CAD build for the part. Positions are in the model's coordinates, mm. A direction names the side the tool comes from. Coordinates: 2 decimals unless noted, no trailing zeros. Loops run counter-clockwise (first coordinate to the right, second up) from the corner with the lowest first, then second, coordinate; pieces in that order, holes last.
1) Pin check, flat tips, straight feed: pin 1 Ø0.8 at (y, z) = (0.5, 18) entering from -X; pin 2 Ø1.3 at (y, z) = (1, 6.5) entering from +X; pin 3 Ø0.8 at (x, y) = (-6, 1) entering from +Z. Stop position of each tip, or through.
2) Two-plate mould, pull along Y, no slides. Class faces 1 (the cylindrical face through (-21.197, -7.24, 12.522)), 2 (the flat face through (-21.374, 1, 19)), 3 (the cylindrical face through (-5.85, -8.62, 12.52)), 4 (the flat face through (-6, 1.588, 6)): +Y half, -Y half, draft (parallel to the pull), parting line (faces both ways), or undercut.
3) Saw through at C-C, the plane y = -6.35. Write the cut outline in (x, z).
4) Which spindle directions (+Z, -Z, +X, -X, +Y, -Y) get a long thin tool onto all of the face, cutting with end or side? Do faces 5 (the flat face through (-19, 1, 4.026)), 6 (the flat face through (-6, 1, 8.674)), 7 (the flat face through (-16.726, 1, 6)), 8 (the flat face through (-4.026, 1, 19)), 9 (the flat face through (-21.374, 1, 6)). Say none if no direction does.
5) Saw through at A-A, the plane z = 12.7. Write the cut outline in (x, y).
6) Wall check: line 1 along X through (y, z) = (-6.5, 16); line 2 along Y through (x, z) = (-6.35, 12.25); line 3 along X through (y, z) = (-5.5, 13.5). Give the ranges that are in metal, low to high.
7) Saw through at B-B, the plane x = -12.7. Write the cut outline in (y, z).
8) Saw through at D-D, the plane y = 0.5. Write the cut outline in (x, z).
Autodesk Inventor part; units mm, degrees
ref_plane "YZ Plane" through (0, 0, 0) normal (1, 0, 0) x (0, 1, 0)
ref_plane "XZ Plane" through (0, 0, 0) normal (0, 1, 0) x (-1, 0, 0)
ref_plane "XY Plane" through (0, 0, 0) normal (0, 0, 1) x (1, 0, 0)
sketch "Sketch1" plane through (0, 0, 0) normal (0, 1, 0) x (-1, 0, 0)
  line L0 (0, 0) -> (25.4, 0)
  line L1 (25.4, 0) -> (25.4, 25.4)
  line L2 (25.4, 25.4) -> (0, 25.4)
  line L3 (0, 25.4) -> (0, 0)
  line L4 (12.7, 25.4) -> (12.7, 0)
  line L5 (12.7, 25.4) -> (38.1, 25.4) construction
  line L6 (0, 12.7) -> (25.4, 12.7)
  line L7 (0, 12.7) -> (25.4, 12.7) construction
  line L8 (12.7, 6.35) -> (25.4, 6.35)
  line L9 (12.7, 6.35) -> (25.4, 6.35) construction
  line L10 (19.05, 0) -> (19.05, 12.7)
  line L11 (16.7259, 16.7259) -> (21.3741, 16.7259)
  line L12 (21.3741, 16.7259) -> (21.3741, 21.3741)
  line L13 (21.3741, 21.3741) -> (16.7259, 21.3741)
  line L14 (16.7259, 21.3741) -> (16.7259, 16.7259)
  line L15 (16.7259, 16.7259) -> (19.05, 19.05) construction
  line L16 (21.3741, 16.7259) -> (16.7259, 21.3741) construction
  line L17 (8.6741, 16.7259) -> (8.6741, 21.3741)
  line L18 (8.6741, 21.3741) -> (4.0259, 21.3741)
  line L19 (4.0259, 21.3741) -> (4.0259, 16.7259)
  line L20 (4.0259, 16.7259) -> (8.6741, 16.7259)
  line L21 (21.3741, 4.0259) -> (21.3741, 8.6741)
  line L22 (21.3741, 8.6741) -> (16.7259, 8.6741)
  line L23 (16.7259, 8.6741) -> (16.7259, 4.0259)
  line L24 (16.7259, 4.0259) -> (21.3741, 4.0259)
  line L25 (8.6741, 4.0259) -> (8.6741, 8.6741)
  line L26 (8.6741, 8.6741) -> (4.0259, 8.6741)
  line L27 (4.0259, 8.6741) -> (4.0259, 4.0259)
  line L28 (4.0259, 4.0259) -> (8.6741, 4.0259)
  circle A0 centre (12.7, 12.7) radius 2.3241
  dimension "d0" = 25.4
  dimension "d1" = 25.4
  dimension "d2" = 25.4
  dimension "d3" = 90
  dimension "d4" = 25.4
  dimension "d5" = 0
  dimension "d6" = 12.7
  dimension "d7" = 0
  dimension "d8" = 4.6482
  dimension "d9" = 4.6482
  dimension "d12" = 12.7
  dimension "d15" = 12.7
  dimension "d18" = 4.6482
extrude "Extrusion1" add sketch "Sketch1" along normal blind 1.5875 contours L24 L23 L8 L10 | L10 L8 L21 L24 | L23 L22 L10 L8 | L10 L22 L21 L8 | L14 L13 L12 L11 | L20 L19 L18 L17 | L28 L27 L26 L25
extrude "Extrusion2" add sketch "Sketch1" against normal blind 10.668 contours L3 L6 A0 L4 L0 | L4 L8 L23 L24 L10 L0 | L3 L2 L4 A0 L6 | L10 L24 L21 L8 L1 L0 | L4 A0 L6 L10 L22 L23 L8 | A0 L4 L6 | L6 L4 A0 | L24 L23 L8 L10 | L10 L8 L21 L24 | L4 L6 A0 | L23 L22 L10 L8 | L2 L1 L6 A0 L4 | L4 A0 L6 | L8 L21 L22 L10 L6 L1 | L10 L22 L21 L8 | L14 L13 L12 L11 | L20 L19 L18 L17 | L28 L27 L26 L25
hole "Hole1" at (-12.7, 0, 12.7) direction (0, -1, 0) diameter 4.6482 depth 32.3342 tip angle 118
sketch "Sketch2" plane through (0, 0, 0) normal (0, 0, -1) x (-1, 0, 0)
  line L0 (25.4, 0) -> (0, 0)
  line L1 (25.4, 0) -> (0, 0)
  line L2 (12.7, 2.032) -> (12.7, -10.668)
  line L3 (15.0241, -10.668) -> (10.3759, -10.668)
  line L4 (12.7, -5.334) -> (25.4, -5.334)
  line L5 (25.4, 0) -> (25.4, -10.668)
  line L6 (12.7, -5.334) -> (0, -5.334)
  line L7 (0, 0) -> (0, -10.668)
  circle A0 centre (19.05, -6.35) radius 2.3241
  circle A1 centre (6.35, -6.35) radius 2.3241
  dimension "d30" = 4.6482
extrude "Extrusion3" cut sketch "Sketch2" against normal through all contours A0 L4 | L4 A0 | A1 L6 | L6 A1
properties part number "odom connector"
Data:
1. pin 1: stops at x = -21.37
1. pin 2: stops at x = -4.03
1. pin 3: stops at z = 21.37
2. face 1: undercut
2. face 2: draft
2. face 3: undercut
2. face 4: +Y half
3. outline: (-25.4, 0) - (-21.37, 0) - (-21.37, 25.4) - (-25.4, 25.4) - close; (-16.73, 0) - (-8.67, 0) - (-8.67, 25.4) - (-16.73, 25.4) - close; (-4.03, 0) - (0, 0) - (0, 25.4) - (-4.03, 25.4) - close; hole circle Ø4.65 at (-12.7, 12.7)
4. face 5: -Z, +X, -X, +Y
4. face 6: +X, -X, +Y
4. face 7: +Z, -Z, +Y
4. face 8: +Z, -Z, +X, +Y
4. face 9: +Z, -Z, -X, +Y
5. outline: (-25.4, -10.67) - (-15.02, -10.67) - (-15.02, 0) - (-25.4, 0) - close; (-10.38, -10.67) - (0, -10.67) - (0, 0) - (-10.38, 0) - close; hole circle Ø4.65 at (-19.05, -6.35); hole circle Ø4.65 at (-6.35, -6.35)
6. line 1: x = -25.4 to -21.37, -16.73 to -8.67, -4.03 to 0
6. line 2: y = -10.67 to -8.67, -4.03 to 0
6. line 3: x = -25.4 to -21.21, -16.89 to -14.88, -10.52 to -8.51, -4.19 to 0
7. outline: (-10.67, 0) - (0, 0) - (0, 10.38) - (-10.67, 10.38) - close; (-10.67, 15.02) - (0, 15.02) - (0, 25.4) - (-10.67, 25.4) - close
8. outline: (-21.37, 4.03) - (-16.73, 4.03) - (-16.73, 8.67) - (-21.37, 8.67) - close; (-21.37, 16.73) - (-16.73, 16.73) - (-16.73, 21.37) - (-21.37, 21.37) - close; (-8.67, 4.03) - (-4.03, 4.03) - (-4.03, 8.67) - (-8.67, 8.67) - close; (-8.67, 16.73) - (-4.03, 16.73) - (-4.03, 21.37) - (-8.67, 21.37) - close
